Verification items for the finished model (mm, model axes). Round coordinates to 2 decimals unless told otherwise and drop trailing zeros. Write each loop counter-clockwise with the first axis right and the second up, starting at its lowest first coordinate (ties: lowest second). Pieces come first, ordered by that corner, then holes. Notation, with made-up numbers: (-4.5, -24) - (32.5, -24) arc R29 ccw to (32.5, 1) - close; hole circle Ø7 at (63, -1). An arc over 180 degrees is marked (long way). Answer as a JSON object with one key per item and string values.
Autodesk Inventor part; units mm, degrees
ref_plane "YZ Plane" through (0, 0, 0) normal (1, 0, 0) x (0, 1, 0)
ref_plane "XZ Plane" through (0, 0, 0) normal (0, 1, 0) x (-1, 0, 0)
ref_plane "XY Plane" through (0, 0, 0) normal (0, 0, 1) x (1, 0, 0)
sketch "Sketch1" plane through (0, 0, 0) normal (0, 0, 1) x (1, 0, 0)
  circle A0 centre (0, 0) radius 7.5
  line L0 (-1.7809, 3.0847) -> (1.7809, 3.0847)
  line L1 (0, 0) -> (3.1, 0) construction
  line L2 (0, 0) -> (1.55, 2.6847) construction
  line L3 (0, 0) -> (-1.55, 2.6847) construction
  line L4 (0, 0) -> (-3.1, 0) construction
  line L5 (0, 0) -> (-1.55, -2.6847) construction
  line L6 (0, 0) -> (1.55, -2.6847) construction
  line L7 (-1.55, 2.6847) -> (1.55, 2.6847)
  line L8 (1.55, 2.6847) -> (3.1, 0)
  line L9 (3.1, 0) -> (1.55, -2.6847)
  line L10 (1.55, -2.6847) -> (-1.55, -2.6847)
  line L11 (-1.55, -2.6847) -> (-3.1, 0)
  line L12 (-3.1, 0) -> (-1.55, 2.6847)
  dimension "d0" = 3.1
  dimension "d3" = 360
extrude "Extrusion1" add sketch "Sketch1" against normal blind 95 contours L7 L8 L9 L10 L11 L12
sketch "Sketch2" plane through (-1.55, 2.6847, 0) normal (0, 1, 0) x (1, 0, 0)
  line L0 (0, 0) -> (0, 95)
  line L1 (3.1, 0) -> (3.1, 95)
  circle A0 centre (1.55, 33.9) radius 0.65
  circle A1 centre (1.55, 36.9) radius 0.65
  line L2 (3.1, 0) -> (0, 0)
  circle A2 centre (1.5476, 33.9) radius 0.65
  circle A3 centre (1.55, 90) radius 0.65
  line L3 (0, 95) -> (3.1, 95)
  point P0 (1.55, 0)
  point P1 (1.55, 0)
  point P2 (1.55, 0)
  point P3 (1.5488, 34.55)
  point P4 (1.5488, 33.25)
  dimension "d7" = 1.3
  dimension "d8" = 3
  dimension "d9" = 33.9
  dimension "d10" = 5
extrude "Extrusion2" cut sketch "Sketch2" against normal blind 10 contours A0 A2 | A2 A0 | A1 | A3
properties part number "eje4_n"
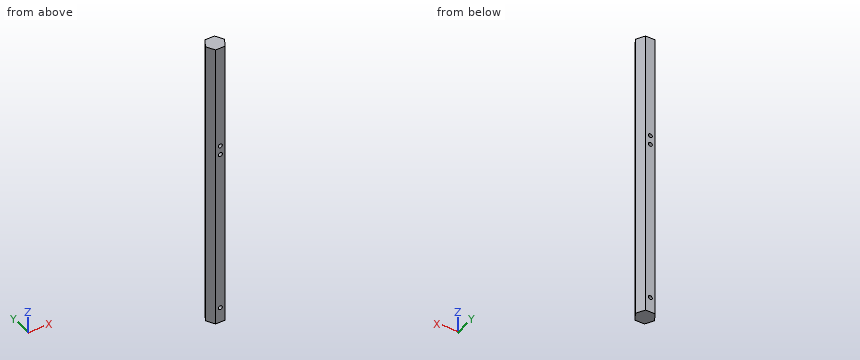
Q1. Gauge pin test, flat end, axial feed: P1, Ø3, axis at y = -2, z = -24.5, coming from the +X side. Record the tip position at first contact, or that the pin passes through.
Geometry check:
{"P1": "stops at x = 2.81"}
Q2. Material ranges on line 1 along Z through (x, y) = (0, -0.8); line 2 along X through (y, z) = (0.75, -49.5); line 3 along X through (y, z) = (1.45, -36.9), recorded low to high. Write a range as [from, to].
Geometry check:
{"line 1": "z = [-95, -90.65], [-89.35, -37.55], [-36.25, -34.55], [-33.25, 0]", "line 2": "x = [-2.67, 2.67]", "line 3": "x = [-2.26, -0.65], [0.65, 2.26]"}
Q3. Section check A-A, the plane y = -1.35. Record the cut outline in (x, z).
Geometry check:
{"outline": "(-2.32, -95) - (2.32, -95) - (2.32, 0) - (-2.32, 0) - close; hole circle Ø1.3 at (0, -90); hole circle Ø1.3 at (0, -36.9); hole circle Ø1.3 at (0, -33.9)"}
Q4. Section check B-B, the plane z = -77.5. Record the cut outline in (x, y).
Geometry check:
{"outline": "(-3.1, 0) - (-1.55, -2.68) - (1.55, -2.68) - (3.1, 0) - (1.55, 2.68) - (-1.55, 2.68) - close"}
